Verification items for the finished model (mm, model axes). A direction names the side the tool comes from. Coordinates: 2 decimals unless noted, no trailing zeros. Order: outer loops, then holes, each group sorted by start corner. A loop starts at its lowest first (then second) coordinate and runs counter-clockwise, first axis right, second up. Notation, with made-up numbers: M 1.5,61 L 33.5,61 A29 cw 33.5,84 Z; hole C 2,-19.5 d2. An arc over 180 degrees is marked long. Return JSON: item names as keys, results as strings. Group by question number.
1. Material ranges on line 1 along Y through (x, z) = (-15.5, -5.85); line 2 along X through (y, z) = (15, -5); line 3 along Y through (x, z) = (-4.5, 18), recorded low to high.
2. Gauge pin test, flat ends, axial feed: pin 1 (15 mm diameter, centred on x = -5, z = 9, fed in from +Y); pin 2 (15 mm diameter, centred on y = 1.5, z = 10, fed in from -X); pin 3 (8 mm diameter, centred on y = 16.5, z = 6, fed in from -X); pin 4 (5 mm diameter, centred on x = -2.5, z = 22.5, fed in from +Y). Record the tip position at first contact, or that the pin passes through.
3. Mould release check, pull along X, two halves, no side actions. Record for faces 1 (the cylindrical face through (-14, -15.43, -5.28)), 2 (the flat face through (-16, -16, 9)), 3 (the flat face through (18.6, -18.7, -3.7)): +X half, -X half, draft (parallel to the pull), parting line (faces both ways), or undercut.
4. Set-up check for faces 4 (the flat face through (0, -21, 9)), 5 (the flat face through (20.15, 0, 31)), 6 (the flat face through (-15, 16, -3)), 7 (the flat face through (-17.912, 17.974, 30.937)), 8 (the flat face through (7.5, 24, 21)): record each of +Z, -Z, +X, -X, +Y, -Y from which the full face is reachable in a straight line by a thin tool's end or side.
5. Section check A-A, the plane y = 13. Record the cut outline in (x, z).
6. Section check B-B, the plane z = 28. Record the cut outline in (x, y).
7. Section check C-C, the plane x = -12.5. Record the cut outline in (y, z), plus the area to 3 significant figures.
```python
from build123d import *

# Parameters (mm, degrees)
SKETCH_1_W          = 42
SKETCH_1_H          = 42
EXTRUDE_1_DEPTH     = 19
CHAMFER_1_SIZE      = 10
SKETCH_2_W          = 42.3
SKETCH_2_H          = 42.3
EXTRUDE_2_DEPTH     = 7.5
SKETCH_3_W          = 42.3
SKETCH_3_H          = 42.3
EXTRUDE_3_DEPTH     = 7.5
CHAMFER_2_SIZE      = 5
SKETCH_4_R          = 1.5
CUT_EXTRUDE_1_DEPTH = 4.5
SKETCH_5_R          = 11
SKETCH_5_R_2        = 3.75
EXTRUDE_4_DEPTH     = 2
SKETCH_6_R          = 2.5
EXTRUDE_5_DEPTH     = 24
CUT_EXTRUDE_START   = -19
CUT_EXTRUDE_2_DEPTH = 19
CHAMFER_3_SIZE      = 0.5
EXTRUDE_6_DEPTH     = 2.5
FILLET_1_R          = 1
EXTRUDE_7_DEPTH     = 5
EXTRUDE_8_DEPTH     = 9
CHAMFER_4_SIZE      = 2.5


with BuildPart() as part:
    # 草图1 → 凸台-拉伸1 (new body)
    with BuildSketch(Plane.XY):
        Rectangle(SKETCH_1_W, SKETCH_1_H)
    extrude(amount=EXTRUDE_1_DEPTH)

    # 倒角1
    chamfer_1_edges = [part.edges().sort_by_distance(p)[0] for p in [
        (21, -21, 9.5),
        (-21, -21, 9.5),
        (-21, 21, 9.5),
        (21, 21, 9.5),
    ]]
    chamfer(chamfer_1_edges, length=CHAMFER_1_SIZE)

    # 草图2 → 凸台-拉伸2 (add)
    with BuildSketch(Plane.XY.offset(19)):
        Rectangle(SKETCH_2_W, SKETCH_2_H)
    extrude(amount=EXTRUDE_2_DEPTH)

    # 草图3 → 凸台-拉伸3 (add)
    with BuildSketch(Plane(origin=(0, 0, 0), x_dir=(-1, 0, 0), z_dir=(0, 0, -1))):
        Rectangle(SKETCH_3_W, SKETCH_3_H)
    extrude(amount=EXTRUDE_3_DEPTH)

    # 倒角2
    chamfer_2_edges = [part.edges().sort_by_distance(p)[0] for p in [
        (21.15, -21.15, 22.75),
        (21.15, 21.15, 22.75),
        (-21.15, 21.15, 22.75),
        (-21.15, -21.15, 22.75),
        (-21.15, -21.15, -3.75),
        (-21.15, 21.15, -3.75),
        (21.15, 21.15, -3.75),
        (21.15, -21.15, -3.75),
    ]]
    chamfer(chamfer_2_edges, length=CHAMFER_2_SIZE)

    # 草图4 → 切除-拉伸1 (cut)
    with BuildSketch(Plane(origin=(0, 0, -7.5), x_dir=(-1, 0, 0), z_dir=(0, 0, -1))):
        with Locations((-15.5, 15.5)):
            Circle(SKETCH_4_R)
        with Locations((15.5, 15.5)):
            Circle(SKETCH_4_R)
        with Locations((15.5, -15.5)):
            Circle(SKETCH_4_R)
        with Locations((-15.5, -15.5)):
            Circle(SKETCH_4_R)
    extrude(amount=-CUT_EXTRUDE_1_DEPTH, mode=Mode.SUBTRACT)

    # 草图5 → 凸台-拉伸4 (add)
    with BuildSketch(Plane(origin=(0, 0, -7.5), x_dir=(-1, 0, 0), z_dir=(0, 0, -1))):
        Circle(SKETCH_5_R)
        Circle(SKETCH_5_R_2, mode=Mode.SUBTRACT)
    extrude(amount=EXTRUDE_4_DEPTH)

    # 草图6 → 凸台-拉伸5 (add)
    with BuildSketch(Plane(origin=(0, 0, -7.5), x_dir=(-1, 0, 0), z_dir=(0, 0, -1))):
        Circle(SKETCH_6_R)
    extrude(amount=EXTRUDE_5_DEPTH)

    # 草图7 → 切除-拉伸2 (cut)
    with BuildSketch(Plane(origin=(0, 0, -31.5), x_dir=(-1, 0, 0), z_dir=(0, 0, -1)).offset(CUT_EXTRUDE_START)):
        with BuildLine():
            Line((2, 1.5), (-2, 1.5))
            ThreePointArc((-2, 1.5), (0, 2.5), (2, 1.5))
        make_face()
    extrude(amount=CUT_EXTRUDE_2_DEPTH, mode=Mode.SUBTRACT)

    # 倒角3
    chamfer_3_edges = [part.edges().sort_by_distance(p)[0] for p in [
        (0.790569415, -2.371708245, -31.5),
    ]]
    chamfer(chamfer_3_edges, length=CHAMFER_3_SIZE)

    # 草图8 → 凸台-拉伸6 (add)
    with BuildSketch(Plane.XY.offset(26.5)):
        Polygon((0, 21.15), (-8, 21.15), (-8, 25.15), (8, 25.15), (8, 21.15), align=None)
    extrude(amount=-EXTRUDE_6_DEPTH)

    # 圆角1
    fillet_1_edges = [part.edges().sort_by_distance(p)[0] for p in [
        (-12.075, 21.15, 26.5),
        (8, 23.15, 26.5),
        (0, 25.15, 26.5),
        (-8, 23.15, 26.5),
        (0, -21.15, 26.5),
        (-21.15, 0, 26.5),
        (21.15, 0, 26.5),
        (12.075, 21.15, 26.5),
        (-18.65, 18.65, 26.5),
        (18.65, 18.65, 26.5),
        (18.65, -18.65, 26.5),
        (-18.65, -18.65, 26.5),
    ]]
    fillet(fillet_1_edges, radius=FILLET_1_R)

    # 草图9 → 凸台-拉伸7 (add)
    with BuildSketch(Plane(origin=(0, 21.15, 0), x_dir=(1, 0, 0), z_dir=(0, 1, 0))):
        Polygon((7.9, -19), (5, -19), (5, -19.5), (7.5, -19.5), (7.5, -23.5), (-7.5, -23.5), (-7.5, -19.5), (-5, -19.5), (-5, -19), (-7.9, -19), (-7.9, -24), (7.9, -24), align=None)
    extrude(amount=EXTRUDE_7_DEPTH)

    # 草图10 → 凸台-拉伸8 (add)
    with BuildSketch(Plane.XY.offset(26.5)):
        Polygon((-7, 20.15), (-15.735786438, 20.15), (-20.15, 15.735786438), (-20.15, -15.735786438), (-15.735786438, -20.15), (15.735786438, -20.15), (20.15, -15.735786438), (20.15, 15.735786438), (15.735786438, 20.15), (7, 20.15), (7, 24.15), (-7, 24.15), align=None)
    extrude(amount=EXTRUDE_8_DEPTH)

    # 倒角4
    # the kernel refuses this chamfer: 2.5 mm, written as the material it adds along each edge
    with BuildSketch(Plane(origin=(0, 0, -7.5), x_dir=(-1, 0, 0), z_dir=(0, -1, 0))) as chamfer_4_piece_1:
        Polygon((2.5 + CHAMFER_4_SIZE, 0), (2.5, CHAMFER_4_SIZE), (2.5, 0), align=None)
    revolve(axis=Axis((0, 0, -7.5), (0, 0, -1)))


solid = part.part
```
Answers follow:
{
 "1": {"line 1": "-21.15 to -17, -14 to 14, 17 to 21.15", "line 2": "-21.15 to -16.91, -14.09 to 14.09, 16.91 to 21.15", "line 3": "-21 to 21"},
 "2": {"pin 1": "y = 21", "pin 2": "x = -21", "pin 3": "x = -19.5", "pin 4": "y = 26.15"},
 "3": {"face 1": "undercut", "face 2": "-X half", "face 3": "+X half"},
 "4": {"face 4": "+X, -X, -Y", "face 5": "+Z, +X, +Y, -Y", "face 6": "-Z", "face 7": "+Z, -X, +Y", "face 8": "+Y"},
 "5": {"outline": "M -21.15,-7.5 L 21.15,-7.5 L 21.15,0 L 19,0 L 19,19 L 21.15,19 L 21.15,25.5 A1 ccw 20.15,26.5 L 20.15,35.5 L -20.15,35.5 L -20.15,26.5 A1 ccw -21.15,25.5 L -21.15,19 L -19,19 L -19,0 L -21.15,0 Z"},
 "6": {"outline": "M -20.15,-15.74 L -15.74,-20.15 L 15.74,-20.15 L 20.15,-15.74 L 20.15,15.74 L 15.74,20.15 L 7,20.15 L 7,24.15 L -7,24.15 L -7,20.15 L -15.74,20.15 L -20.15,15.74 Z"},
 "7": {"outline": "M -21.15,-7.5 L 21.15,-7.5 L 21.15,0 L 19.5,0 L 19.5,19 L 21.15,19 L 21.15,25.5 A1 ccw 20.15,26.5 L 20.15,35.5 L -20.15,35.5 L -20.15,26.5 A1 ccw -21.15,25.5 L -21.15,19 L -19.5,19 L -19.5,0 L -21.15,0 Z", "area": "1,740 mm^2"}
}
